Design review of the part built by this model. Coordinates are the model's own, in mm. Face numbers are marked on the shaded views. A direction names the side the tool comes from. Give positions to 0.01 mm unless a question says otherwise; leave off trailing zeros. Order: outer loops, then holes, each group sorted by start corner. A loop starts at its lowest first (then second) coordinate and runs counter-clockwise, first axis right, second up. Notation, with made-up numbers: (43, 3) -> (62, 3) arc R23 ccw to (62, 22) -> close; hole circle Ø6 at (-11.75, 84.5). An arc over 180 degrees is marked (long way). One line per item, written item: value.
from build123d import *

# Parameters (mm, degrees)
F0_R      = 25
F1_DEPTH  = 30
F0_W      = 90
F0_H      = 94
F2_DEPTH  = 25
F3_SIZE   = 4.99999
F4_W      = 25.1866029114
F4_H      = 31.7543679761
F5_DEPTH  = 100
F6_DEPTH  = 100
F7_W      = 30
F7_H      = 15
F8_DEPTH  = 1000
F9_W      = 20
F9_H      = 15
F10_DEPTH = 100


# Not quite as in the source:
# - a fillet or chamfer is up to 0.001 mm smaller than in the source, because OpenCascade refuses the exact size


with BuildPart() as f1:
    # F0 (on Top) → F1 (new body)
    with BuildSketch(Plane.XY):
        with Locations((16.9619322568, -28.2926298678)):
            Circle(F0_R)
    extrude(amount=F1_DEPTH)

    # F0 (on Top) → F2 (join)
    with BuildSketch(Plane.XY):
        with Locations((16.9619322568, -28.2926298678)):
            Rectangle(F0_W, F0_H)
        with Locations((16.9619322568, -28.2926298678)):
            Circle(F0_R, mode=Mode.SUBTRACT)
    extrude(amount=F2_DEPTH)

    # F3 (size 5 in the source; OpenCascade refuses exactly that, so slightly less here)
    f3_edges = [f1.edges().sort_by_distance(p)[0] for p in [
        (-8.038068, -28.29263, 30),
    ]]
    chamfer(f3_edges, length=F3_SIZE)

    # F4 (on face) → F5 (cut)
    with BuildSketch(Plane.XY.offset(25)):
        with Locations((49.3686308011, 2.8301861442)):
            Rectangle(F4_W, F4_H)
    extrude(amount=-F5_DEPTH, mode=Mode.SUBTRACT)

    # F4 (on face) → F6 (cut)
    with BuildSketch(Plane.XY.offset(25)):
        with Locations((-15.4447662875, 2.8301861442)):
            Rectangle(F4_W, F4_H)
        with Locations((-15.4447662875, -59.4154458798)):
            Rectangle(F4_W, F4_H)
        with Locations((49.3686308011, -59.4154458798)):
            Rectangle(F4_W, F4_H)
    extrude(amount=-F6_DEPTH, mode=Mode.SUBTRACT)

    # F7 (on face) → F8 (cut)
    with BuildSketch(Plane(origin=(0, 18.7073701322, 0), x_dir=(-1, 0, 0), z_dir=(0, 1, 0))):
        with Locations((-16.7753293454, 12.5)):
            Rectangle(F7_W, F7_H)
    extrude(amount=-F8_DEPTH, mode=Mode.SUBTRACT)

    # F9 (on face) → F10 (cut)
    with BuildSketch(Plane.YZ.offset(61.9619322568)):
        with Locations((-27.5469978439, 12.5)):
            Rectangle(F9_W, F9_H)
    extrude(amount=-F10_DEPTH, mode=Mode.SUBTRACT)


solid = f1.part
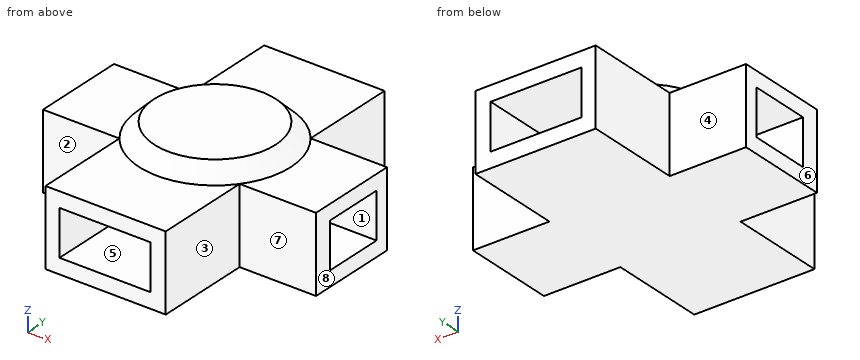
Item 1: Add section D-D on z = 27. Give the boundary of the cut face in (x, y), plus the area to 3 significant figures.
Returned:
outline: circle Ø46 at (16.96, -28.29)
area: 1,660 mm²
Item 2: Machinability: for the marked faces 1, 2, 3 and 4, which of the approach directions +Z, -Z, +X, -X, +Y, -Y give a long, thin tool a straight path to every point of the face, cutting with its end or side? Answer none if there is none.
Returned:
face 1: +X, -X
face 2: +Z, -Z, -X, -Y
face 3: +Z, -Z, +X, -Y
face 4: +Z, -Z, -X, +Y
Item 3: Add section A-A on x = -15. Give the boundary of the cut face in (y, z).
Returned:
outline: (-43.54, 0) -> (-13.05, 0) -> (-13.05, 25) -> (-43.54, 25) -> close; hole (-37.55, 5) -> (-17.55, 5) -> (-17.55, 20) -> (-37.55, 20) -> close
Item 4: Draft analysis for pull direction X (two halves, no side actions). For the marked faces 5, 6, 7 and 8, state which applies: pulls with the +X half, pulls with the -X half, needs draft (parallel to the pull), parting line crosses it, or undercut.
Returned:
face 5: undercut
face 6: pulls with the -X half
face 7: needs draft
face 8: pulls with the +X half
Item 5: Add section B-B on z = 7.25. Give the boundary of the cut face in (x, y), plus the area to 3 significant figures.
Returned:
outline: (-28.04, -43.54) -> (-2.85, -43.54) -> (-2.85, -75.29) -> (1.78, -75.29) -> (1.78, -37.55) -> (-28.04, -37.55) -> close; (-28.04, -17.55) -> (1.78, -17.55) -> (1.78, 18.71) -> (-2.85, 18.71) -> (-2.85, -13.05) -> (-28.04, -13.05) -> close; (31.78, -75.29) -> (36.78, -75.29) -> (36.78, -43.54) -> (61.96, -43.54) -> (61.96, -37.55) -> (31.78, -37.55) -> close; (31.78, -17.55) -> (61.96, -17.55) -> (61.96, -13.05) -> (36.78, -13.05) -> (36.78, 18.71) -> (31.78, 18.71) -> close
area: 1,240 mm²
Item 6: Clearance check with flat-ended pins moving along their axes: P1, Ø4.5, axis at x = 47.5, z = 11, coming from the +Y side; P2, Ø1, axis at y = -6.5, z = 14.5, coming from the +X side; P3, Ø12, axis at x = -15, z = 12.5, coming from the -Y side. State where each tip first meets the part, or that it passes through.
Returned:
P1: y = -13.05
P2: x = 36.78
P3: y = -43.54
Item 7: Add section C-C on y = -65.5. Give the boundary of the cut face in (x, z).
Returned:
outline: (-2.85, 0) -> (36.78, 0) -> (36.78, 25) -> (-2.85, 25) -> close; hole (1.78, 5) -> (31.78, 5) -> (31.78, 20) -> (1.78, 20) -> close
Item 8: To check wall thickness, follow line 1 along Y through (x, z) = (-0.5, 13.25); line 2 along Z through (x, y) = (15.5, -25.5); line 3 along Y through (x, z) = (-14.5, 9). State the ranges of each line that lie inside material, in increasing order. Write a range as from..to.
Returned:
line 1: -75.29..-37.55, -17.55..18.71
line 2: 0..5, 20..30
line 3: -43.54..-37.55, -17.55..-13.05
